Geometry check sheet. Reference: the model listing, model coordinates, mm. Give positions to 0.01 mm unless a question says otherwise; leave off trailing zeros. Loops run counter-clockwise (first coordinate to the right, second up) from the corner with the lowest first, then second, coordinate; pieces in that order, holes last. Notation, with made-up numbers: (25.25, 84) -> (44.25, 84) arc R16 cw to (44.25, 97) -> close; hole circle Ø9 at (-21.75, 64.5). An arc over 180 degrees is marked (long way). Write each question's results on one line, items separated by ' | '. Start each with the question number.
1) Sectioned sample at B-B on z = 129. Record the cut outline in (x, y), then the cut area to 3 significant figures.
2) Sectioned sample at A-A on x = 0. Record the cut outline in (y, z).
3) Scan lines: line 1 (Y direction, x = 62, z = -359.5); line 2 (Z direction, x = -1, y = 3.5); line 3 (Z direction, x = 0, y = -6). Record each from-to range of solid material in increasing order. Write a range as from..to.
4) Sectioned sample at C-C on x = -301.5. Record the cut outline in (y, z), then the cut area to 3 significant figures.
5) Depth check by flat-ended pin: pin 1 (6 mm diameter, centred on y = 12.5, z = -226.5, fed in from -X); pin 2 (3 mm diameter, centred on x = -56.5, y = 15.5, fed in from -Z); pin 3 (4 mm diameter, centred on x = -84, z = -246.5, fed in from +Y). Enter the tip coordinate at first touch or a pass-through.
```python
from build123d import *

# Parameters (mm, degrees)
BOSS_EXTRUDE1_DEPTH    = 30
SKETCH4_W              = 1518.677694458
SKETCH4_H              = 842.1
BOSS_EXTRUDE2_DEPTH    = 11.1125
F_20_0MM_DOWEL_HOLE1_D = 101.6
SKETCH8_W              = 1.5875
SKETCH8_H              = 30
BOSS_EXTRUDE3_DEPTH    = 269.05
CUT_EXTRUDE1_DEPTH     = 1021.368996981


with BuildPart() as part:
    # Sketch3 → Boss-Extrude1 (new body)
    with BuildSketch(Plane(origin=(0, 0, 0), x_dir=(1, 0, 0), z_dir=(0, 1, 0))):
        with BuildLine():
            Line((-524, 0), (-525.5875, 0))
            ThreePointArc((-525.5875, 0), (-255.243310314, 459.448661655), (277.677694458, 446.248045549))
            Line((277.677694458, 446.248045549), (277.677694458, 444.377202386))
            ThreePointArc((277.677694458, 444.377202386), (-254.040241009, 458.300726541), (-524, 0))
        make_face()
    extrude(amount=BOSS_EXTRUDE1_DEPTH)

    # Sketch4 → Boss-Extrude2 (add)
    with BuildSketch(Plane(origin=(0, 0, 0), x_dir=(1, 0, 0), z_dir=(0, 1, 0))):
        with Locations((-88.661152771, 145.65)):
            Rectangle(SKETCH4_W, SKETCH4_H)
    extrude(amount=-BOSS_EXTRUDE2_DEPTH)

    # Ø20.0mm Dowel Hole1 (through all)
    with Locations(Plane(origin=(0, 0, 0), x_dir=(1, 0, 0), z_dir=(0, 1, 0))):
        with Locations((0, 0)):
            Hole(F_20_0MM_DOWEL_HOLE1_D / 2)

    # Sketch8 → Boss-Extrude3 (add)
    with BuildSketch(Plane.XY):
        with Locations((-524.79375, 15)):
            Rectangle(SKETCH8_W, SKETCH8_H)
    extrude(amount=BOSS_EXTRUDE3_DEPTH)

    # Sketch9 → Cut-Extrude1 (cut, through all)
    with BuildSketch(Plane(origin=(0, 0, 0), x_dir=(1, 0, 0), z_dir=(0, 1, 0))):
        Polygon((270.669120675, 346.737850878), (92.835706926, 397.730761704), (84.566586251, 368.892910826), (262.4, 317.9), align=None)
    extrude(amount=-CUT_EXTRUDE1_DEPTH, mode=Mode.SUBTRACT)


solid = part.part
```
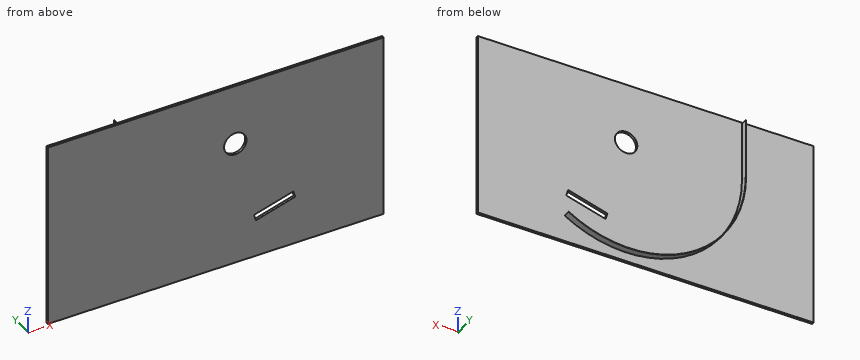
Result:
1) outline: (-848, -11.11) -> (670.68, -11.11) -> (670.68, 0) -> (-524, 0) -> (-524, 30) -> (-525.59, 30) -> (-525.59, 0) -> (-848, 0) -> close | area: 16,900 mm^2
2) outline: (-11.11, -566.7) -> (0, -566.7) -> (0, -525.59) -> (30, -525.59) -> (30, -524) -> (0, -524) -> (0, -50.8) -> (-11.11, -50.8) -> close; (-11.11, 50.8) -> (0, 50.8) -> (0, 275.4) -> (-11.11, 275.4) -> close
3) line 1: -11.11..0 | line 2: -525.59..-524 | line 3: -566.7..-50.8, 50.8..275.4
4) outline: (-11.11, -566.7) -> (0, -566.7) -> (0, -430.51) -> (30, -430.51) -> (30, -428.57) -> (0, -428.57) -> (0, 275.4) -> (-11.11, 275.4) -> close | area: 9,420 mm^2
5) pin 1: x = -475.7 | pin 2: z = -522.7 | pin 3: y = 0
